Work out the finished part from the listing and answer in its coordinate system (mm). Round coordinates to 2 decimals unless told otherwise and drop trailing zeros. Loops run counter-clockwise (first coordinate to the right, second up) from the corner with the lowest first, then second, coordinate; pieces in that order, holes last.
from build123d import *

# Parameters (mm, degrees)
F0_W     = 698.5
F0_H     = 635
F1_DEPTH = 10.16
F4_DEPTH = 10.161
F5_R     = 5.07999
F6_R     = 5.07999
F8_D     = 15.24


# Not quite as in the source:
# - a fillet or chamfer is up to 0.001 mm smaller than in the source, because OpenCascade refuses the exact size


with BuildPart() as f1:
    # F0 (on Front) → F1 (new body)
    with BuildSketch(Plane.XZ):
        with Locations((349.25, 317.5)):
            Rectangle(F0_W, F0_H)
    extrude(amount=F1_DEPTH)

    # F3 (on face) → F4 (cut, through all)
    with BuildSketch(Plane(origin=(0, 0, 0), x_dir=(-1, 0, 0), z_dir=(0, 1, 0))):
        with BuildLine():
            Line((-25.4, 190.5), (-25.4, 444.5))
            ThreePointArc((-25.4, 444.5), (-50.8, 469.9), (-76.2, 444.5))
            Line((-76.2, 444.5), (-76.2, 190.5))
            ThreePointArc((-76.2, 190.5), (-50.8, 165.1), (-25.4, 190.5))
        make_face()
    extrude(amount=-F4_DEPTH, mode=Mode.SUBTRACT)

    # F5 (radius 5.08 in the source; OpenCascade refuses exactly that, so slightly less here)
    f5_edges = [f1.edges().sort_by_distance(p)[0] for p in [
        (50.8, 0, 165.1),
        (76.2, -10.16, 317.5),
    ]]
    fillet(f5_edges, radius=F5_R)

    # F6 (radius 5.08 in the source; OpenCascade refuses exactly that, so slightly less here)
    f6_edges = [f1.edges().sort_by_distance(p)[0] for p in [
        (349.25, -10.16, 635),
        (349.25, 0, 635),
        (349.25, -10.16, 0),
        (349.25, 0, 0),
    ]]
    fillet(f6_edges, radius=F6_R)

    # F8 (through all)
    with Locations(Plane.XZ.offset(10.16)):
        with Locations((496.1636, 528.32), (331.0636, 528.32), (661.2636, 528.32), (661.2636, 106.68), (496.1636, 106.68), (331.0636, 106.68)):
            Hole(F8_D / 2)


solid = f1.part
Item 1: Determine the mould class of faces 1 (the face through (344, -10.16, 322)), 2 (the face through (653.995, -5.009, 108.969)) for opening direction Z: pulls with the +Z half, pulls with the -Z half, needs draft (parallel to the pull), parting line crosses it, or undercut.
Item 2: This flat-tipped pin is pushed along its axis until it touches: P1, Ø1, axis at x = 428, z = 179.5, coming from the +Y side. Where does it stop, or does it pass through?
Item 3: Section B-B, the plane y = -6.75 is taken. Give the vertices of the cut face in (x, z).
Item 4: Section C-C, the plane z = 106.68 is taken. Give the vertices of the cut face in (x, y).
Item 5: Straight lines are drawn through the part: line 1 (X direction, y = -2.5, z = 528.32); line 2 (Z direction, x = 337, y = -3); line 3 (X direction, y = -4.75, z = 447.5). For each, find the intervals that lie inside material, in ascending order.
Answer below:
1. face 1: needs draft
1. face 2: undercut
2. P1: stops at y = 0
3. outline: (0, 0.28) - (698.5, 0.28) - (698.5, 634.72) - (0, 634.72) - close; hole (25.12, 190.5) arc R25.68 ccw to (76.48, 190.5) - (76.48, 444.5) arc R25.68 ccw to (25.12, 444.5) - close; hole circle Ø15.24 at (331.06, 106.68); hole circle Ø15.24 at (331.06, 528.32); hole circle Ø15.24 at (496.16, 106.68); hole circle Ø15.24 at (496.16, 528.32); hole circle Ø15.24 at (661.26, 106.68); hole circle Ø15.24 at (661.26, 528.32)
4. outline: (0, -10.16) - (323.44, -10.16) - (323.44, 0) - (0, 0) - close; (338.68, -10.16) - (488.54, -10.16) - (488.54, 0) - (338.68, 0) - close; (503.78, -10.16) - (653.64, -10.16) - (653.64, 0) - (503.78, 0) - close; (668.88, -10.16) - (698.5, -10.16) - (698.5, 0) - (668.88, 0) - close
5. line 1: x = 0 to 323.44, 338.68 to 488.54, 503.78 to 653.64, 668.88 to 698.5
5. line 2: z = 0.45 to 101.9, 111.46 to 523.54, 533.1 to 634.55
5. line 3: x = 0 to 25.57, 76.03 to 698.5
